```python
from build123d import *

# Parameters (mm, degrees)
F1_DEPTH = 9
F2_T     = -3
F3_R     = 2.99999


# Not quite as in the source:
# - a fillet or chamfer is up to 0.001 mm smaller than in the source, because OpenCascade refuses the exact size


with BuildPart() as f1:
    # F0 (on Top) → F1 (new body)
    with BuildSketch(Plane.XY):
        with BuildLine():
            Line((-74.3585927405, 75.2026882768), (-74.3585927405, -53.5473117232))
            Line((-74.3585927405, -53.5473117232), (-2.3585927405, -53.5473117232))
            Line((-2.3585927405, -53.5473117232), (-2.3585927405, 75.2026882768))
            ThreePointArc((-2.3585927405, 75.2026882768), (-4.189175358, 79.6221056592), (-8.6085927405, 81.4526882768))
            Line((-8.6085927405, 81.4526882768), (-68.1085927405, 81.4526882768))
            ThreePointArc((-68.1085927405, 81.4526882768), (-72.5280101229, 79.6221056592), (-74.3585927405, 75.2026882768))
        make_face()
    extrude(amount=F1_DEPTH)

    # F2
    f2_openings = [f1.faces().sort_by_distance(p)[0] for p in [
        (-38.358593, 13.83847, 9),
    ]]
    offset(amount=F2_T, openings=f2_openings)

    # F3 (radius 3 in the source; OpenCascade refuses exactly that, so slightly less here)
    f3_edges = [f1.edges().sort_by_distance(p)[0] for p in [
        (-38.358593, -53.547312, 9),
    ]]
    fillet(f3_edges, radius=F3_R)


solid = f1.part
```
Design review of the part built by this model. Coordinates are the model's own, in mm. A direction names the side the tool comes from. Coordinates: 2 decimals unless noted, no trailing zeros. Order: outer loops, then holes, each group sorted by start corner. A loop starts at its lowest first (then second) coordinate and runs counter-clockwise, first axis right, second up. Notation, with made-up numbers: M 6.5,10 L 31.5,10 A26 cw 31.5,27 Z; hole C 18,5 d11. An arc over 180 degrees is marked long. Answer as a JSON object with one key per item and string values. Group by question number.
1) Wall thickness on L1, parallel to X at y = -43, z = 8.25; L2, parallel to Y at x = -8.5, z = 6.25; L3, parallel to Z at x = -34.5, y = -42.5: over which ranges is each line inside the solid? List them lowest first.
2) Add section C-C, the plane z = 7.5. Write out the cut boundary in (x, y).
3) Tool access review of faces 4 (the flat face through (-39, -50.547, 6)), 5 (the flat face through (-2.359, 10, 4)): name each direction out of +Z, -Z, +X, -X, +Y, -Y from which nothing blocks a thin tool from reaching the whole face with its end or side.
4) Add section B-B, the plane y = -1.5. Write out the cut boundary in (x, z), then the cut area to 3 significant figures.
5) Mouldability with a two-part tool opening along Y and no side actions: class faces 1 (the flat face through (-38, 78.453, 6)), 2 (the flat face through (-39, 15, 0)), 3 (the cylindrical face through (-72.48, 79.67, 4.44)) as pulls with the +Y half, pulls with the -Y half, needs draft (parallel to the pull), parting line crosses it, or undercut.
6) For pin 1 (1 mm diameter, centred on x = -42.5, y = 31.5, fed in from -Z); pin 2 (4 mm diameter, centred on x = -45.5, y = 47, fed in from +Z), all flat-tipped, find the tip position at first contact; note any pin that passes through.
Computed values:
{
 "1": {"L1": "x = -74.36 to -71.36, -5.36 to -2.36", "L2": "y = -53.54 to -50.55, 78.45 to 81.45", "L3": "z = 0 to 3"},
 "2": {"outline": "M -74.36,-53.15 L -2.36,-53.15 L -2.36,75.2 A6.25 ccw -8.61,81.45 L -68.11,81.45 A6.25 ccw -74.36,75.2 Z; hole M -71.36,-50.55 L -5.36,-50.55 L -5.36,75.2 A3.25 ccw -8.61,78.45 L -68.11,78.45 A3.25 ccw -71.36,75.2 Z"},
 "3": {"face 4": "+Z", "face 5": "+Z, -Z, +X, +Y, -Y"},
 "4": {"outline": "M -74.36,0 L -2.36,0 L -2.36,9 L -5.36,9 L -5.36,3 L -71.36,3 L -71.36,9 L -74.36,9 Z", "area": "252 mm^2"},
 "5": {"face 1": "undercut", "face 2": "needs draft", "face 3": "pulls with the +Y half"},
 "6": {"pin 1": "stops at z = 0", "pin 2": "stops at z = 3"}
}
